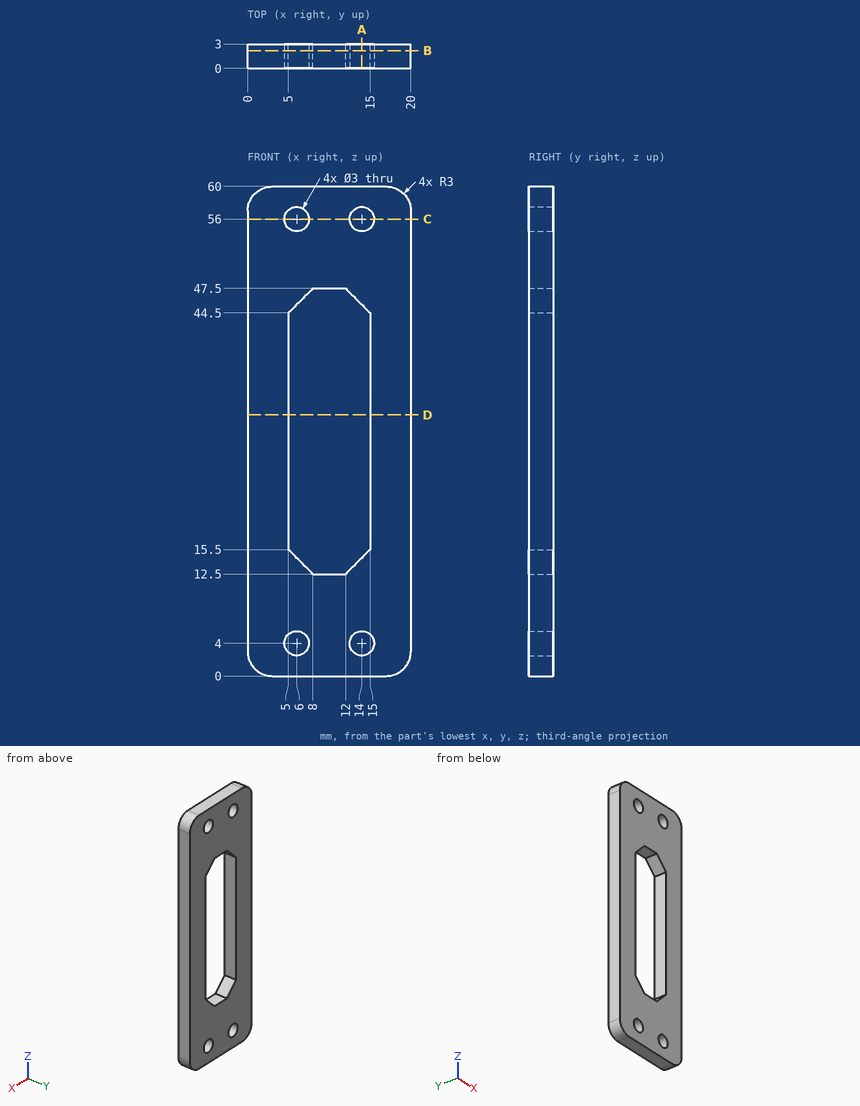
Verification items for this drawing (mm, ordinates from the low corner). Round coordinates to 2 decimals unless told otherwise and drop trailing zeros. Order: outer loops, then holes, each group sorted by start corner. A loop starts at its lowest first (then second) coordinate and runs counter-clockwise, first axis right, second up. Notation, with made-up numbers: M 45.25,-15.75 L 81.25,-15.75 A16 cw 81.25,0.25 Z; hole C -5,-35.5 d9. An arc over 180 degrees is marked long. Answer in a Markdown table with one row per item. Add a question column.
Item 1: Material ranges on L1, parallel to X at y = 1.2, z = 4; L2, parallel to Z at x = 10.25, y = 1.3; L3, parallel to Z at x = 15.25, y = 2, recorded low to high. Write a range as [from, to].
Item 2: Sectioned sample at D-D, the plane z = 32. Enter the section's corners in (x, y), plus the area to 3 significant figures.
Item 3: Sectioned sample at A-A, the plane x = 14. Enter the section's corners in (y, z).
Item 4: Sectioned sample at B-B, the plane y = 2.2. Enter the section's corners in (x, z).
Item 5: Sectioned sample at C-C, the plane z = 56. Enter the section's corners in (x, y), plus the area to 3 significant figures.
Filled in:
| question | item | result |
|---|---|---|
| 1 | L1 | x = [0, 4.5], [7.5, 12.5], [15.5, 20] |
| 1 | L2 | z = [0, 12.5], [47.5, 60] |
| 1 | L3 | z = [0, 3.17], [4.83, 55.17], [56.83, 60] |
| 2 | outline | M 0,0 L 5,0 L 5,3 L 0,3 Z; M 15,0 L 20,0 L 20,3 L 15,3 Z |
| 2 | area | 30.0 mm² |
| 3 | outline | M 0,0 L 3,0 L 3,2.5 L 0,2.5 Z; M 0,5.5 L 3,5.5 L 3,14.5 L 0,14.5 Z; M 0,45.5 L 3,45.5 L 3,54.5 L 0,54.5 Z; M 0,57.5 L 3,57.5 L 3,60 L 0,60 Z |
| 4 | outline | M 0,3 A3 ccw 3,0 L 17,0 A3 ccw 20,3 L 20,57 A3 ccw 17,60 L 3,60 A3 ccw 0,57 Z; hole C 6,4 d3; hole C 6,56 d3; hole M 5,15.5 L 8,12.5 L 12,12.5 L 15,15.5 L 15,44.5 L 12,47.5 L 8,47.5 L 5,44.5 Z; hole C 14,4 d3; hole C 14,56 d3 |
| 5 | outline | M 0,0 L 4.5,0 L 4.5,3 L 0,3 Z; M 7.5,0 L 12.5,0 L 12.5,3 L 7.5,3 Z; M 15.5,0 L 20,0 L 20,3 L 15.5,3 Z |
| 5 | area | 42.0 mm² |
